from build123d import *

# Parameters (mm, degrees)
SKETCH1_R           = 7.25
BOSS_EXTRUDE1_DEPTH = 1
CHAMFER1_SIZE       = 0.5
SKETCH2_W           = 1.2
SKETCH2_H           = 11
BOSS_EXTRUDE2_DEPTH = 3
SKETCH3_R           = 9.45
BOSS_EXTRUDE3_DEPTH = 1.2
SKETCH4_W           = 0.85
SKETCH4_H           = 18
BOSS_EXTRUDE4_DEPTH = 100
CIRPATTERN2_COUNT   = 2
CIRPATTERN2_ANGLE   = 90
SKETCH6_R           = 11
BOSS_EXTRUDE5_DEPTH = 1.5


with BuildPart() as part:
    # Sketch1 → Boss-Extrude1 (new body)
    with BuildSketch(Plane(origin=(0, 0, 0), x_dir=(1, 0, 0), z_dir=(0, 1, 0))):
        with Locations(Location((0, 0, 0), (0, 0, 270))):
            Circle(SKETCH1_R)
    extrude(amount=BOSS_EXTRUDE1_DEPTH)

    # Chamfer1
    chamfer1_edges = [part.edges().sort_by_distance(p)[0] for p in [
        (0, 0, -7.25),
    ]]
    chamfer(chamfer1_edges, length=CHAMFER1_SIZE)

    # Sketch2 → Boss-Extrude2 (add)
    with BuildSketch(Plane(origin=(0, 1, 0), x_dir=(1, 0, 0), z_dir=(0, 1, 0))):
        Rectangle(SKETCH2_W, SKETCH2_H)
    boss_extrude2 = extrude(amount=BOSS_EXTRUDE2_DEPTH)

    # Sketch3 → Boss-Extrude3 (add)
    with BuildSketch(Plane(origin=(0, 4, 0), x_dir=(1, 0, 0), z_dir=(0, 1, 0))):
        with Locations(Location((0, 0, 0), (0, 0, 270))):
            Circle(SKETCH3_R)
    extrude(amount=BOSS_EXTRUDE3_DEPTH)

    # Sketch4 → Boss-Extrude4 (add)
    with BuildSketch(Plane(origin=(0, 5.2, 0), x_dir=(1, 0, 0), z_dir=(0, 1, 0))):
        Rectangle(SKETCH4_W, SKETCH4_H)
    boss_extrude4 = extrude(amount=BOSS_EXTRUDE4_DEPTH)

    # CirPattern2: Boss-Extrude2, Boss-Extrude4 ×2 about axis
    cirpattern2_axis = Axis((0, 0, 0), (0, 1, 0))
    add([boss_extrude2.rotate(cirpattern2_axis, i * CIRPATTERN2_ANGLE / (CIRPATTERN2_COUNT - 1)) for i in range(1, CIRPATTERN2_COUNT)])
    add([boss_extrude4.rotate(cirpattern2_axis, i * CIRPATTERN2_ANGLE / (CIRPATTERN2_COUNT - 1)) for i in range(1, CIRPATTERN2_COUNT)])

    # Sketch6 → Boss-Extrude5 (add)
    with BuildSketch(Plane(origin=(0, 105.2, 0), x_dir=(1, 0, 0), z_dir=(0, 1, 0))):
        with Locations(Location((0, 0, 0), (0, 0, 270))):
            Circle(SKETCH6_R)
    extrude(amount=BOSS_EXTRUDE5_DEPTH)


solid = part.part
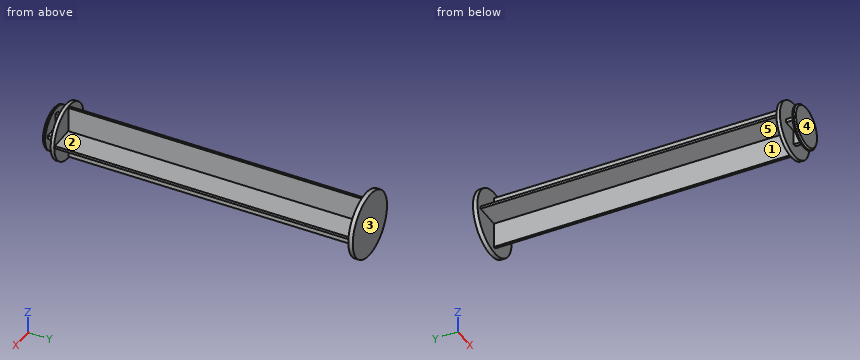
Input: part model. Units: mm. Frame: model coordinates. Face numbers are marked on the shaded views. A direction names the side the tool comes from. Coordinates: 2 decimals unless noted, no trailing zeros. Loops run counter-clockwise (first coordinate to the right, second up) from the corner with the lowest first, then second, coordinate; pieces in that order, holes last.
(1) First-contact query: pin 1 Ø3 at (x, y) = (-5.5, 69) entering from +Z (3 decimals); pin 2 Ø1.3 at (x, y) = (0, 2.5) entering from -Z; pin 3 Ø3.5 at (x, y) = (4, 3) entering from -Z. Flat tips, straight axial feed; report the tip coordinate or a pass-through.
(2) Section A-A on y = 42. Return the cut outline in (x, z) (3 decimals).
(3) Set-up query: the marked faces 1 and 2. Return all of +Z, -Z, +X, -X, +Y, -Y with unobstructed straight access to the full face (end or side cutting, diameter ignored); none if empty.
(4) Material intervals for probe 1 along Y at (x, z) = (-0.75, -4.5); probe 2 along Y at (x, z) = (-3, 8.75); probe 3 along Y at (x, z) = (3.25, 6), sorted ascending.
(5) Pull-direction query (Y, two-part tool) for the marked faces 3, 4 and 5; classes: released by +Y, released by -Y, zero draft, split by the parting line, or undercut.
Data:
1. pin 1: stops at z = 0.425
1. pin 2: stops at z = -5.5
1. pin 3: stops at z = -9.1
2. outline: (-9, -0.425) - (-0.425, -0.425) - (-0.425, -9) - (0.425, -9) - (0.425, -0.425) - (9, -0.425) - (9, 0.425) - (0.425, 0.425) - (0.425, 9) - (-0.425, 9) - (-0.425, 0.425) - (-9, 0.425) - close
3. face 1: -Z, -X
3. face 2: +Z, +X
4. probe 1: y = 0 to 1, 4 to 5.2, 105.2 to 106.7
4. probe 2: y = 4 to 5.2, 105.2 to 106.7
4. probe 3: y = 0.07 to 1, 4 to 5.2, 105.2 to 106.7
5. face 3: released by +Y
5. face 4: released by -Y
5. face 5: undercut
